```python
from build123d import *

# Parameters (mm, degrees)
BOSS_EXTRUDE1_DEPTH = 20
SKETCH2_R           = 12.5
BOSS_EXTRUDE2_DEPTH = 10
SKETCH3_R           = 12.5
BOSS_EXTRUDE3_DEPTH = 20
SKETCH4_R           = 12.5
BOSS_EXTRUDE6_DEPTH = 88.9
SKETCH6_R           = 12.5
BOSS_EXTRUDE7_DEPTH = 15


with BuildPart() as part:
    # Sketch1 → Boss-Extrude1 (new body)
    with BuildSketch(Plane(origin=(0, 0, 0), x_dir=(0, 0, -1), z_dir=(1, 0, 0))):
        with BuildLine():
            ThreePointArc((12.5, 0), (10.155048006, 7.288689869), (4, 11.842719282))
            Line((4, 11.842719282), (4, 9))
            Line((4, 9), (-4, 9))
            Line((-4, 9), (-4, 11.842719282))
            ThreePointArc((-4, 11.842719282), (-7.288689869, -10.155048006), (12.5, 0))
        make_face()
    extrude(amount=BOSS_EXTRUDE1_DEPTH)

    # Sketch2 → Boss-Extrude2 (add)
    with BuildSketch(Plane(origin=(20, 0, 0), x_dir=(0, 0, -1), z_dir=(1, 0, 0))):
        with Locations(Location((0, 0, 0), (0, 0, 108.662924885))):
            Circle(SKETCH2_R)
    extrude(amount=BOSS_EXTRUDE2_DEPTH)

    # Sketch3 → Boss-Extrude3 (add)
    with BuildSketch(Plane(origin=(30, 0, 0), x_dir=(0, 0, -1), z_dir=(1, 0, 0))):
        with Locations(Location((0, 0, 0), (0, 0, 108.662924885))):
            Circle(SKETCH3_R)
    extrude(amount=BOSS_EXTRUDE3_DEPTH)

    # Sketch4 → Boss-Extrude6 (add)
    with BuildSketch(Plane(origin=(50, 0, 0), x_dir=(0, 0, -1), z_dir=(1, 0, 0))):
        with BuildLine():
            ThreePointArc((17.5, 0), (14.0312152, 10.458250332), (5, 16.770509831))
            Line((5, 16.770509831), (5, 13.5))
            Line((5, 13.5), (-5, 13.5))
            Line((-5, 13.5), (-5, 16.770509831))
            ThreePointArc((-5, 16.770509831), (-10.458250332, -14.0312152), (17.5, 0))
        make_face()
        with Locations(Location((0, 0, 0), (0, 0, 108.662924885))):
            Circle(SKETCH4_R, mode=Mode.SUBTRACT)
        with Locations(Location((0, 0, 0), (0, 0, 108.662924885))):
            Circle(SKETCH4_R)
    extrude(amount=BOSS_EXTRUDE6_DEPTH)

    # Sketch6 → Boss-Extrude7 (add)
    with BuildSketch(Plane(origin=(138.9, 0, 0), x_dir=(0, 0, -1), z_dir=(1, 0, 0))):
        with Locations(Location((0, 0, 0), (0, 0, 108.662924885))):
            Circle(SKETCH6_R)
    extrude(amount=BOSS_EXTRUDE7_DEPTH)


solid = part.part
```
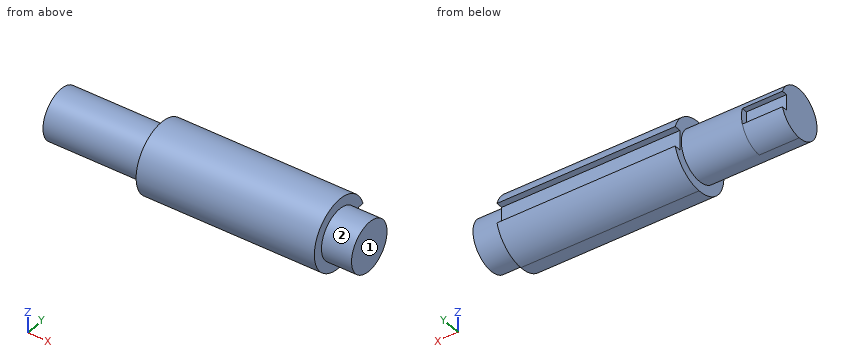
The listing builds one solid part. Answer for the finished solid, in the listing's coordinates (mm). Face numbers are marked on the shaded views. A direction names the side the tool comes from. Give positions to 0.01 mm unless a question says otherwise; leave off trailing zeros. Write each loop counter-clockwise with the first axis right and the second up, starting at its lowest first coordinate (ties: lowest second). Pieces come first, ordered by that corner, then holes. Notation, with made-up numbers: (37, -5) - (79, -5) arc R13 cw to (79, 12) - close; hole circle Ø10 at (-16.75, 52). An arc over 180 degrees is marked (long way). Use one line per item in the form item = value. Start each with the question number.
1) Find section D-D on z = -14. Determine the outline of the cut face in (x, y), plus the area to 3 significant figures.
2) Find section B-B on x = 119. Determine the outline of the cut face in (y, z).
3) Flat-ended cylindrical pins translate along their axes: pin 1 Ø3 at (x, z) = (34.5, -2) entering from -Y; pin 2 Ø4 at (x, z) = (72, -6) entering from +Y; pin 3 Ø8 at (x, y) = (80, -10.5) entering from +Z. Find the tip coordinate at first contact, or state that the pin passes through.
4) Find section C-C on x = 28.5. Determine the outline of the cut face in (y, z), plus the area to 3 significant figures.
5) A tool of negligible diameter and unlimited length cuts with its end or side. For the marked faces 1 and 2, from which of +Z, -Z, +X, -X, +Y, -Y can it reach the whole face along a straight path? Write none if from no direction.
6) Consider line 1 along X through (y, z) = (-5.5, 11.5); line 2 along Y through (x, z) = (93, 0); line 3 along Z through (x, y) = (69, -1). Determine where each line is inside the solid, lowest interval first. Write a range as from..to.
7) Find section A-A on z = 0. Determine the outline of the cut face in (x, y), plus the area to 3 significant figures.
Geometry results:
q1.outline = (50, -10.5) - (138.9, -10.5) - (138.9, 10.5) - (50, 10.5) - close
q1.area = 1,870 mm2
q2.outline = (13.5, -5) - (13.5, 5) - (16.77, 5) arc R17.5 ccw (long way) to (16.77, -5) - close
q3.pin_1 = -12.49
q3.pin_2 = 16.77
q3.pin_3 = 16.25
q4.outline = circle Ø25 at (0, 0)
q4.area = 491 mm2
q5.face_1 = +Z, -Z, +X, +Y, -Y
q5.face_2 = +X
q6.line_1 = 50..138.9
q6.line_2 = -17.5..13.5
q6.line_3 = -17.47..17.47
q7.outline = (0, -12.5) - (50, -12.5) - (50, -17.5) - (138.9, -17.5) - (138.9, -12.5) - (153.9, -12.5) - (153.9, 12.5) - (138.9, 12.5) - (138.9, 13.5) - (50, 13.5) - (50, 12.5) - (20, 12.5) - (20, 9) - (0, 9) - close
q7.area = 4,310 mm2
